from build123d import *

# Parameters (mm, degrees)
BOSS_EXTRUDE1_DEPTH = 3.175
CUT_EXTRUDE4_START  = 3.175
SKETCH1_4_R         = 12.7
CUT_EXTRUDE4_DEPTH  = 0.79375


with BuildPart() as part:
    # Sketch1 → Boss-Extrude1 (new body)
    with BuildSketch(Plane(origin=(0, 0, 0), x_dir=(1, 0, 0), z_dir=(0, 1, 0))):
        with BuildLine():
            Line((-80.321852568, 0), (-43.18, 0))
            ThreePointArc((-43.18, 0), (-39.587897552, -1.487897552), (-38.1, -5.08))
            Line((-38.1, -5.08), (-38.1, -7.62))
            ThreePointArc((-38.1, -7.62), (-36.612102448, -11.212102448), (-33.02, -12.7))
            Line((-33.02, -12.7), (33.02, -12.7))
            ThreePointArc((33.02, -12.7), (36.612102448, -11.212102448), (38.1, -7.62))
            Line((38.1, -7.62), (38.1, -5.08))
            ThreePointArc((38.1, -5.08), (39.587897552, -1.487897552), (43.18, 0))
            Line((43.18, 0), (80.321852568, 0))
            ThreePointArc((80.321852568, 0), (112.522229673, 17.734693366), (114.745503669, 54.428571429))
            ThreePointArc((114.745503669, 54.428571429), (0, 127), (-114.745503669, 54.428571429))
            ThreePointArc((-114.745503669, 54.428571429), (-112.522229673, 17.734693366), (-80.321852568, 0))
        make_face()
        with BuildLine():
            Line((-1.28, 2.14746362), (-1.28, -2.14746362))
            ThreePointArc((-1.28, -2.14746362), (0, -2.5), (1.28, -2.14746362))
            Line((1.28, -2.14746362), (1.28, 2.14746362))
            ThreePointArc((1.28, 2.14746362), (0, 2.5), (-1.28, 2.14746362))
        make_face(mode=Mode.SUBTRACT)
        with BuildLine():
            Line((-17.443731844, 87.171820099), (-6.406874067, 24.578689239))
            ThreePointArc((-6.406874067, 24.578689239), (0, 25.4), (6.406874067, 24.578689239))
            Line((6.406874067, 24.578689239), (17.443731844, 87.171820099))
            ThreePointArc((17.443731844, 87.171820099), (0, 88.9), (-17.443731844, 87.171820099))
        make_face(mode=Mode.SUBTRACT)
        with BuildLine():
            Line((73.974366197, 49.305204044), (21.910101932, 12.849413735))
            ThreePointArc((21.910101932, 12.849413735), (17.960512242, 17.960512242), (12.849413735, 21.910101932))
            Line((12.849413735, 21.910101932), (49.305204044, 73.974366197))
            ThreePointArc((49.305204044, 73.974366197), (62.861792847, 62.861792847), (73.974366197, 49.305204044))
        make_face(mode=Mode.SUBTRACT)
        with BuildLine():
            Line((87.171820099, 17.443731844), (60.268779933, 12.7))
            Line((60.268779933, 12.7), (87.988181024, 12.7))
            ThreePointArc((87.988181024, 12.7), (87.612112441, 15.077392137), (87.171820099, 17.443731844))
        make_face(mode=Mode.SUBTRACT)
        with BuildLine():
            Line((-87.171820099, 17.443731844), (-60.268779933, 12.7))
            Line((-60.268779933, 12.7), (-87.988181024, 12.7))
            ThreePointArc((-87.988181024, 12.7), (-87.612112441, 15.077392137), (-87.171820099, 17.443731844))
        make_face(mode=Mode.SUBTRACT)
        with BuildLine():
            Line((-49.305204044, 73.974366197), (-12.849413735, 21.910101932))
            ThreePointArc((-12.849413735, 21.910101932), (-17.960512242, 17.960512242), (-21.910101932, 12.849413735))
            Line((-21.910101932, 12.849413735), (-73.974366197, 49.305204044))
            ThreePointArc((-73.974366197, 49.305204044), (-62.861792847, 62.861792847), (-49.305204044, 73.974366197))
        make_face(mode=Mode.SUBTRACT)
    extrude(amount=BOSS_EXTRUDE1_DEPTH)

    # Sketch1_4 → Cut-Extrude4 (cut)
    with BuildSketch(Plane(origin=(0, 0, 0), x_dir=(1, 0, 0), z_dir=(0, 1, 0)).offset(CUT_EXTRUDE4_START)):
        with Locations((-41.310676524, 99.732795535)):
            Circle(SKETCH1_4_R)
        with Locations((-99.732795535, 41.310676524)):
            Circle(SKETCH1_4_R)
        with Locations((-76.332177029, 76.332177029)):
            Circle(SKETCH1_4_R)
        with Locations((0, 107.95)):
            Circle(SKETCH1_4_R)
        with Locations((41.310676524, 99.732795535)):
            Circle(SKETCH1_4_R)
        with Locations((76.332177029, 76.332177029)):
            Circle(SKETCH1_4_R)
        with Locations((99.732795535, 41.310676524)):
            Circle(SKETCH1_4_R)
    extrude(amount=-CUT_EXTRUDE4_DEPTH, mode=Mode.SUBTRACT)


solid = part.part
Model file for the job. Use its own axes, mm. A direction names the side the tool comes from. Give positions to 0.01 mm unless a question says otherwise; leave off trailing zeros. Loops run counter-clockwise (first coordinate to the right, second up) from the corner with the lowest first, then second, coordinate; pieces in that order, holes last. Notation, with made-up numbers: (-26.75, 88) -> (-5.75, 88) arc R19 cw to (-5.75, 100) -> close; hole circle Ø9 at (-29.5, 80.25). An arc over 180 degrees is marked (long way). Use a Markdown table: item, result. Add a question column.
(1) Tool access for faces 1 (the cylindrical face through (-36.651, 1.565, 11.172)), 2 (the flat face through (48.307, 1.565, -31.332)), 3 (the cylindrical face through (-54, 2.8, -100.3)): list every direction of +Z, -Z, +X, -X, +Y, -Y with a clear straight run to the whole face (end or side of a thin tool).
(2) Slice it at C-C on z = -107.95. List the corners of the cut face in (x, y) (3 decimals).
(3) Slice it at D-D on x = 78. List the corners of the cut face in (y, z) (1 decimal), and give its area (3 significant figures).
(4) Wall check: line 1 along Z through (x, y) = (4, 2.5); line 2 along X through (y, z) = (2.7, -99); line 3 along X through (y, z) = (2.65, -107.95). Give the ranges that are in metal, low to high.
(5) Mould opens along Z. For faces 4 (the cylindrical face through (98.08, 2.784, -53.903)), 5 (the cylindrical face through (2.005, 1.565, -126.984)), 6 (the cylindrical face through (-112.806, 1.565, -18.191)) say: +Z half, -Z half, draft (parallel to the pull), parting line (faces both ways), or undercut.
(6) Drop flat-ended pins along their axis: pin 1 Ø1 at (x, y) = (57, 2) entering from +Z; pin 2 Ø7.5 at (x, z) = (-76, -71) entering from +Y; pin 3 Ø1.3 at (y, z) = (1, 6.5) entering from -X. Give the stop position or say it passes through.
(7) Slice it at A-A on y = 0.7. Give the number of separate pieces and of enclosed holes in the cut face, and give its area (3 significant figures).
(8) Slice it at B-B on x = -46. List the corners of the cut face in (y, z) (3 decimals).
Filled sheet:
| question | item | result |
|---|---|---|
| 1 | face 1 | +Z, -X, +Y, -Y |
| 1 | face 2 | +Y, -Y |
| 1 | face 3 | +Y |
| 2 | outline | (-66.901, 0) -> (66.901, 0) -> (66.901, 3.175) -> (50.994, 3.175) -> (50.994, 2.381) -> (31.627, 2.381) -> (31.627, 3.175) -> (12.7, 3.175) -> (12.7, 2.381) -> (-12.7, 2.381) -> (-12.7, 3.175) -> (-31.627, 3.175) -> (-31.627, 2.381) -> (-50.994, 2.381) -> (-50.994, 3.175) -> (-66.901, 3.175) -> close |
| 3 | outline | (0, -100.2) -> (3.2, -100.2) -> (3.2, -88.9) -> (2.4, -88.9) -> (2.4, -63.7) -> (3.2, -63.7) -> (3.2, -15.8) -> (0, -15.8) -> close; (0, -12.7) -> (3.2, -12.7) -> (3.2, 0) -> (0, 0) -> close |
| 3 | area | 288 mm2 |
| 4 | line 1 | -126.94 to -120, -95.9 to -88.81, -25.08 to 12.7 |
| 4 | line 2 | -79.55 to -53.99, -28.63 to -9.01, 9.01 to 28.63, 53.99 to 79.55 |
| 4 | line 3 | -66.9 to -50.99, -31.63 to -12.7, 12.7 to 31.63, 50.99 to 66.9 |
| 5 | face 4 | undercut |
| 5 | face 5 | -Z half |
| 5 | face 6 | parting line |
| 6 | pin 1 | z = 0 |
| 6 | pin 2 | y = 2.38 |
| 6 | pin 3 | x = -38.1 |
| 7 | separate pieces | 1 |
| 7 | enclosed holes | 6 |
| 7 | area | 20,400 mm2 |
| 8 | outline | (0, -118.377) -> (3.175, -118.377) -> (3.175, -111.535) -> (2.381, -111.535) -> (2.381, -87.93) -> (3.175, -87.93) -> (3.175, -69.254) -> (0, -69.254) -> close; (0, -29.717) -> (3.175, -29.717) -> (3.175, 0) -> (0, 0) -> close |
